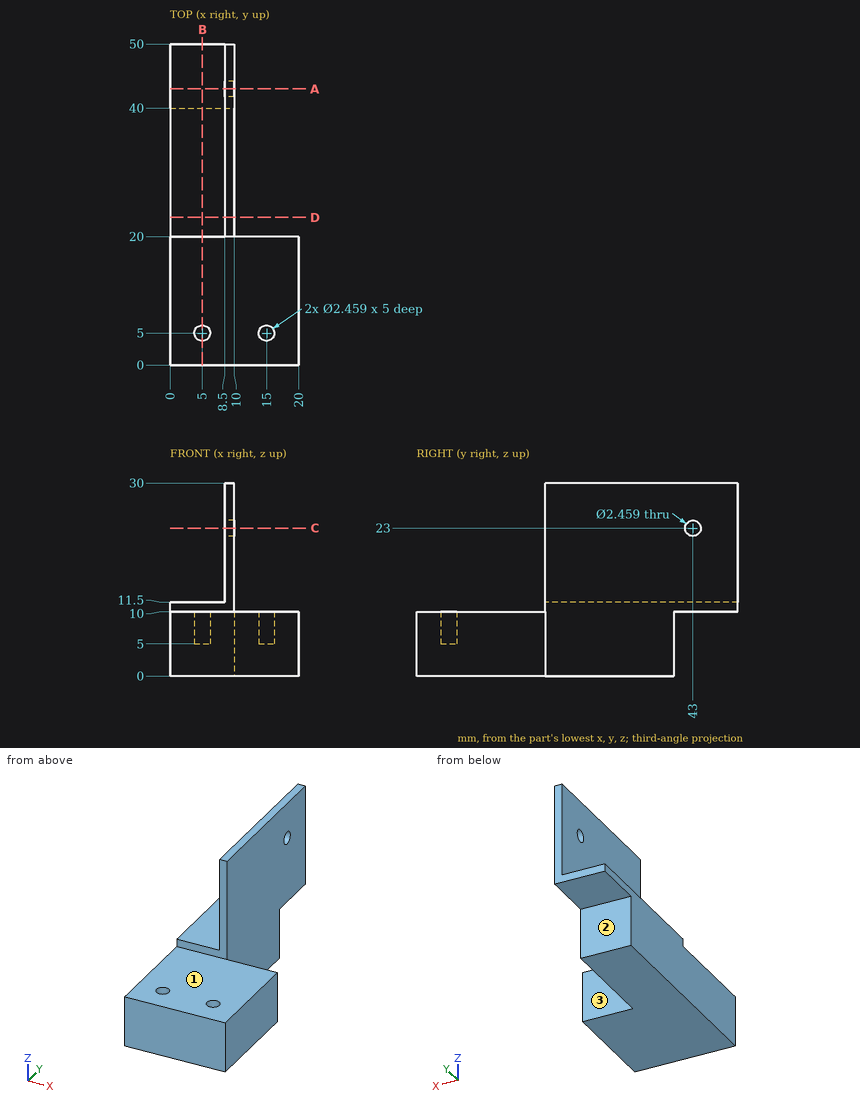
The drawing under review shows one solid part. Ordinate dimensions are in mm from its lowest x, y, z. A direction names the side the tool comes from. Coordinates: 2 decimals unless noted, no trailing zeros. Order: outer loops, then holes, each group sorted by start corner. A loop starts at its lowest first (then second) coordinate and runs counter-clockwise, first axis right, second up. Notation, with made-up numbers: (-1, -8) -> (52, -8) arc R17 cw to (52, 19) -> close; hole circle Ø5 at (29.25, -26.75). An arc over 180 degrees is marked (long way). Answer as CSV lines item,"result".
Q1. Clearance check with flat-ended pins moving along their axes: pin 1 Ø2.5 at (x, y) = (15.5, 5) entering from +Z; pin 2 Ø3 at (x, z) = (17.5, 4.5) entering from +Y; pin 3 Ø2 at (y, z) = (27, 7) entering from +X. State where each tip first meets the part, or that it passes through.
Model answer:
pin 1,"stops at z = 10"
pin 2,"stops at y = 20"
pin 3,"stops at x = 10"
Q2. We need section B-B (x = 5). State the section outline as (y, z) points, plus the area to 3 significant figures.
Model answer:
outline,"(0, 0) -> (40, 0) -> (40, 10) -> (50, 10) -> (50, 11.5) -> (20, 11.5) -> (20, 10) -> (6.23, 10) -> (6.23, 5) -> (3.77, 5) -> (3.77, 10) -> (0, 10) -> close"
area,"433 mm2"
Q3. We need section C-C (z = 23). State the section outline as (x, y) points.
Model answer:
outline,"(8.5, 20) -> (10, 20) -> (10, 41.77) -> (8.5, 41.77) -> close; (8.5, 44.23) -> (10, 44.23) -> (10, 50) -> (8.5, 50) -> close"
Q4. For the marked faces 1, 2 and 3, list the 3-axis set-ups (+Z, -Z, +X, -X, +Y, -Y) from which the entire face can be reached by the end or side of a thin tool; tool diameter is ignored.
Model answer:
face 1,"+Z, +X, -X, -Y"
face 2,"-Z, +X, -X, +Y"
face 3,"+Z, -Z, +X, +Y"
Q5. Wall thickness on line 1 along X through (y, z) = (5, 6.65); line 2 along Y through (x, z) = (5, 6.9); line 3 along Z through (x, y) = (9.1, 43): over which ranges is each line inside the solid? List them lowest first. Write a range as [from, to].
Model answer:
line 1,"x = [0, 3.77], [6.23, 13.77], [16.23, 20]"
line 2,"y = [0, 3.77], [6.23, 40]"
line 3,"z = [10, 21.77], [24.23, 30]"
Q6. We need section A-A (y = 43). State the section outline as (x, z) points.
Model answer:
outline,"(0, 10) -> (10, 10) -> (10, 21.77) -> (8.5, 21.77) -> (8.5, 11.5) -> (0, 11.5) -> close; (8.5, 24.23) -> (10, 24.23) -> (10, 30) -> (8.5, 30) -> close"
Q7. We need section D-D (y = 23). State the section outline as (x, z) points, plus the area to 3 significant figures.
Model answer:
outline,"(0, 0) -> (10, 0) -> (10, 30) -> (8.5, 30) -> (8.5, 11.5) -> (0, 11.5) -> close"
area,"143 mm2"
